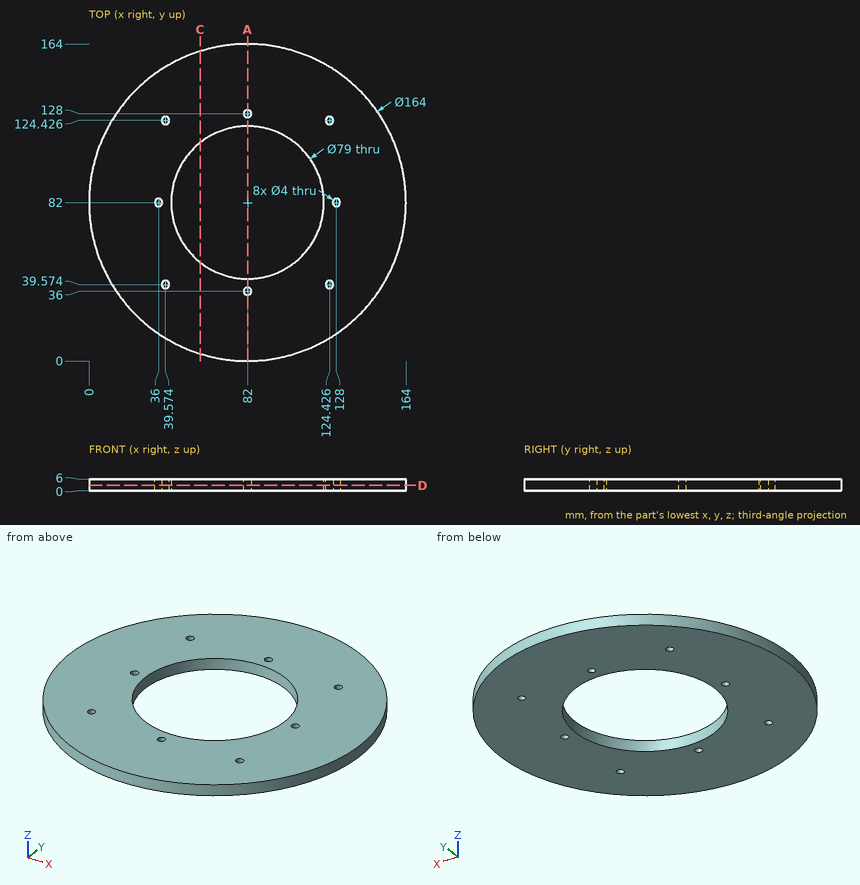
Design review of the part shown in the three views and the two pictorial views. Dimensions are in mm from the part's minimum x, y and z. Round coordinates to 2 decimals unless told otherwise and drop trailing zeros. Loops run counter-clockwise (first coordinate to the right, second up) from the corner with the lowest first, then second, coordinate; pieces in that order, holes last. Notation, with made-up numbers: (73, 19) - (106, 19) arc R19 cw to (106, 35) - close; hole circle Ø3 at (15, -22). An arc over 180 degrees is marked (long way). One line per item, written item: value. Start each with the question number.
Item 1: For L1, parallel to Y at x = 82, z = 4; L2, parallel to X at y = 88.5, z = 2.8; L3, parallel to Y at x = 37.5, z = 4.7 (1 decimal), list the stretches that pass through material, from the lowest coordinate up.
Item 2: Clearance check with flat-ended pins moving along their axes: pin 1 Ø1.5 at (x, z) = (140, 1.5) entering from -Y (1 decimal); pin 2 Ø1.5 at (x, z) = (27.5, 1.5) entering from +Y; pin 3 Ø3 at (y, z) = (99.5, 2) entering from +X. State where each tip first meets the part, or that it passes through.
Item 3: Take a section at A-A (x = 82). Give the boundary of the cut face in (y, z).
Item 4: Take a section at C-C (x = 57.5). Give the boundary of the cut face in (y, z) (1 decimal).
Item 5: Take a section at D-D (z = 2.75). State how many separate pieces and enclosed holes the cut face has, plus the area to 3 significant figures.
Answer below:
1. L1: y = 0 to 34, 38 to 42.5, 121.5 to 126, 130 to 164
1. L2: x = 0.26 to 43.04, 120.96 to 163.74
1. L3: y = 13.1 to 80.7, 83.3 to 150.9
2. pin 1: stops at y = 23.3
2. pin 2: stops at y = 143.93
2. pin 3: stops at x = 162.42
3. outline: (0, 0) - (34, 0) - (34, 6) - (0, 6) - close; (38, 0) - (42.5, 0) - (42.5, 6) - (38, 6) - close; (121.5, 0) - (126, 0) - (126, 6) - (121.5, 6) - close; (130, 0) - (164, 0) - (164, 6) - (130, 6) - close
4. outline: (3.7, 0) - (51, 0) - (51, 6) - (3.7, 6) - close; (113, 0) - (160.3, 0) - (160.3, 6) - (113, 6) - close
5. separate pieces: 1
5. enclosed holes: 9
5. area: 16,100 mm2
